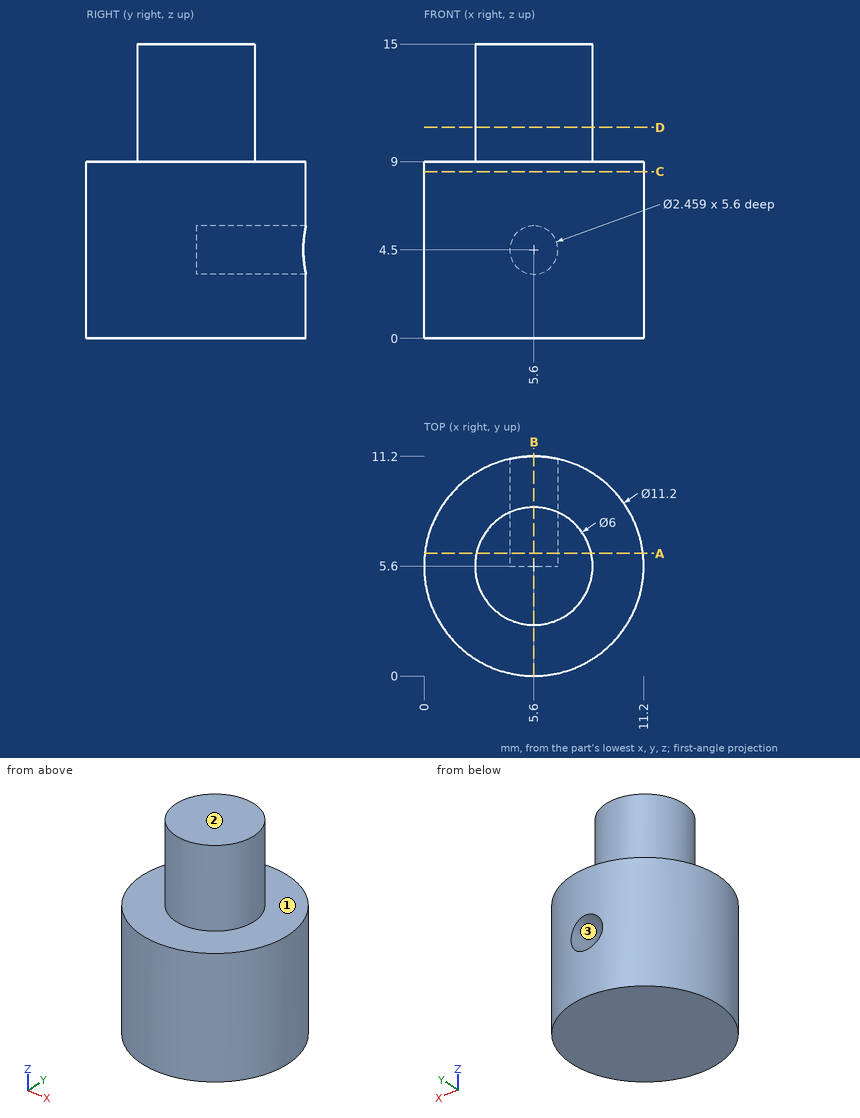
The drawing under review shows one solid part. Ordinate dimensions are in mm from its lowest x, y, z. A direction names the side the tool comes from. Give positions to 0.01 mm unless a question says otherwise; leave off trailing zeros. Write each loop counter-clockwise with the first axis right and the second up, starting at its lowest first coordinate (ties: lowest second). Pieces come first, ordered by that corner, then holes.
1. Add section C-C, the plane z = 8.5. Write out the cut boundary in (x, y), plus the area to 3 significant figures.
2. Add section B-B, the plane x = 5.6. Write out the cut boundary in (y, z), plus the area to 3 significant figures.
3. Tool access review of the marked faces 1, 2 and 3: name each direction out of +Z, -Z, +X, -X, +Y, -Y from which nothing blocks a thin tool from reaching the whole face with its end or side.
4. For P1, Ø3, axis at x = 10, z = 8, coming from the -Y side; P2, Ø6, axis at y = 6, z = 10, coming from the -X side; P3, Ø1.5, axis at y = 2.5, z = 8, coming from the +X side; P4, Ø1, axis at x = 9, y = 3.5, coming from the +Z side, all flat-tipped, find the tip position at first contact; note any pin that passes through.
5. Wall thickness on L1, parallel to Z at x = 1.5, y = 3.25; L2, parallel to Y at x = 5.75, z = 13.25; L3, parallel to X at y = 10.75, z = 3.5: over which ranges is each line inside the solid? List them lowest first.
6. Add section A-A, the plane y = 6.25. Write out the cut boundary in (x, z).
7. Add section D-D, the plane z = 10.75. Write out the cut boundary in (x, y).
Worked answers:
1. outline: circle Ø11.2 at (5.6, 5.6)
1. area: 98.5 mm2
2. outline: (0, 0) - (11.2, 0) - (11.2, 3.27) - (5.6, 3.27) - (5.6, 5.73) - (11.2, 5.73) - (11.2, 9) - (8.6, 9) - (8.6, 15) - (2.6, 15) - (2.6, 9) - (0, 9) - close
2. area: 123 mm2
3. face 1: +Z
3. face 2: +Z, +X, -X, +Y, -Y
3. face 3: +Y
4. P1: stops at y = 0.81
4. P2: stops at x = 0
4. P3: stops at x = 10.68
4. P4: stops at z = 9
5. L1: z = 0 to 9
5. L2: y = 2.6 to 8.6
5. L3: x = 3.4 to 4.88, 6.32 to 7.8
6. outline: (0.04, 0) - (11.16, 0) - (11.16, 9) - (8.53, 9) - (8.53, 15) - (2.67, 15) - (2.67, 9) - (0.04, 9) - close; hole circle Ø2.46 at (5.6, 4.5)
7. outline: circle Ø6 at (5.6, 5.6)
